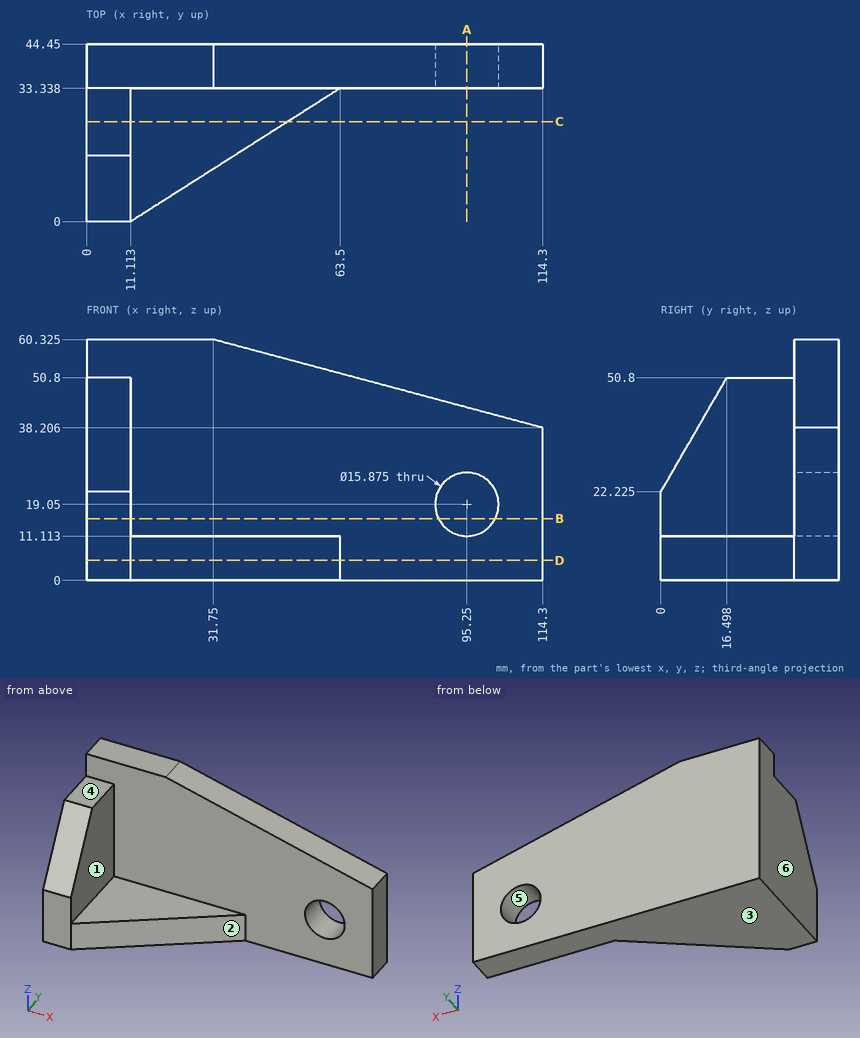
Print and shaded views of the part. All mm, measured from the part's lowest x, y and z. A direction names the side the tool comes from. Give positions to 0.01 mm unless a question says otherwise; leave off trailing zeros. Loops run counter-clockwise (first coordinate to the right, second up) from the corner with the lowest first, then second, coordinate; pieces in that order, holes last. Notation, with made-up numbers: (-29.5, 31) - (25.5, 31) arc R16 cw to (25.5, 55) - close; hole circle Ø8 at (64, -13). An arc over 180 degrees is marked (long way). Use a Markdown table: item, result.
(1) Wall check: line 1 along X through (y, z) = (40, 19); line 2 along Y through (x, z) = (56, 27.5); line 3 along X through (y, z) = (8.5, 28). Give the ranges that are in metal, low to high.
Taken from the geometry:
| item | result |
|---|---|
| line 1 | 0 to 87.31, 103.19 to 114.3 |
| line 2 | 33.34 to 44.45 |
| line 3 | 0 to 11.11 |
(2) Which spindle directions (+Z, -Z, +X, -X, +Y, -Y) get a long thin tool onto all of the face, cutting with end or side? Do the marked faces 1 and 2. Say none if no direction does.
Taken from the geometry:
| item | result |
|---|---|
| face 1 | +Z, +X, -Y |
| face 2 | +Z, -Z, +X, -Y |
(3) Band-saw the part on C-C (y = 25). Give the cut face in (x, z), and give its area (3 significant figures).
Taken from the geometry:
| item | result |
|---|---|
| outline | (0, 0) - (50.4, 0) - (50.4, 11.11) - (11.11, 11.11) - (11.11, 50.8) - (0, 50.8) - close |
| area | 1,000 mm2 |
(4) Pull direction Z, two halves, no side cores. Call the marked faces 3, 4, 5 and 6: +Z half, -Z half, draft (parallel to the pull), parting line (faces both ways), or undercut.
Taken from the geometry:
| item | result |
|---|---|
| face 3 | -Z half |
| face 4 | +Z half |
| face 5 | undercut |
| face 6 | draft |
(5) Band-saw the part on D-D (z = 5). Give the cut face in (x, y), and give its area (3 significant figures).
Taken from the geometry:
| item | result |
|---|---|
| outline | (0, 0) - (11.11, 0) - (63.5, 33.34) - (114.3, 33.34) - (114.3, 44.45) - (0, 44.45) - close |
| area | 2,510 mm2 |
(6) Band-saw the part on A-A (x = 95.25). Give the cut face in (y, z).
Taken from the geometry:
| item | result |
|---|---|
| outline | (33.34, 0) - (44.45, 0) - (44.45, 11.11) - (33.34, 11.11) - close; (33.34, 26.99) - (44.45, 26.99) - (44.45, 43.31) - (33.34, 43.31) - close |
(7) Drop flat-ended pins along their axis: pin 1 Ø5.5 at (x, y) = (5.5, 24.5) entering from +Z; pin 2 Ø4 at (y, z) = (6.5, 16.5) entering from +X; pin 3 Ø18 at (x, z) = (79.5, 35) entering from -Y. Give the stop position or say it passes through.
Taken from the geometry:
| item | result |
|---|---|
| pin 1 | z = 50.8 |
| pin 2 | x = 11.11 |
| pin 3 | y = 33.34 |
(8) Band-saw the part on B-B (z = 15.5). Give the cut face in (x, y), and give its area (3 significant figures).
Taken from the geometry:
| item | result |
|---|---|
| outline | (0, 0) - (11.11, 0) - (11.11, 33.34) - (88.15, 33.34) - (88.15, 44.45) - (0, 44.45) - close; (102.35, 33.34) - (114.3, 33.34) - (114.3, 44.45) - (102.35, 44.45) - close |
| area | 1,480 mm2 |
